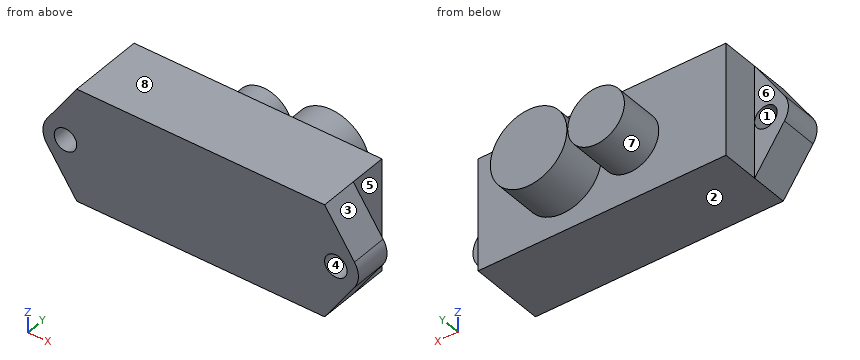
```python
from build123d import *

# Parameters (mm, degrees)
BOSS_EXTRUDE11_DEPTH   = 5
BOSS_EXTRUDE11_2_DEPTH = 5
SKETCH1_5_W            = 33
SKETCH1_5_H            = 15
BOSS_EXTRUDE13_DEPTH   = 10
SKETCH2_R              = 1.5
CUT_EXTRUDE1_DEPTH     = 5
SKETCH3_R              = 3.777846651
BOSS_EXTRUDE18_DEPTH   = 6
SKETCH3_5_R            = 5.1
BOSS_EXTRUDE22_DEPTH   = 6


with BuildPart() as part:
    # Sketch1 → Boss-Extrude11 (new body)
    with BuildSketch(Plane(origin=(0, 0, 0), x_dir=(1, 0, 0), z_dir=(0, 1, 0))):
        with BuildLine():
            Line((-20.475239861, 1.695047972), (-16.5, 7.5))
            Line((-16.5, 7.5), (-16.5, -7.5))
            Line((-16.5, -7.5), (-20.475239861, -1.695047972))
            ThreePointArc((-20.475239861, -1.695047972), (-21, 0), (-20.475239861, 1.695047972))
        make_face()
    extrude(amount=BOSS_EXTRUDE11_DEPTH)



with BuildPart() as body_2:
    # Sketch1 → Boss-Extrude11 2 (new body)
    with BuildSketch(Plane(origin=(0, 0, 0), x_dir=(1, 0, 0), z_dir=(0, 1, 0))):
        with BuildLine():
            ThreePointArc((20.475239861, 1.695047972), (21, 0), (20.475239861, -1.695047972))
            Line((20.475239861, -1.695047972), (16.5, -7.5))
            Line((16.5, -7.5), (16.5, 7.5))
            Line((16.5, 7.5), (20.475239861, 1.695047972))
        make_face()
    extrude(amount=BOSS_EXTRUDE11_2_DEPTH)


with BuildPart() as part_1:
    add(part.part)

    add(body_2.part)  # Boss-Extrude13 merges body 2
    # Sketch1_5 → Boss-Extrude13 (add)
    with BuildSketch(Plane(origin=(0, 0, 0), x_dir=(1, 0, 0), z_dir=(0, 1, 0))):
        Rectangle(SKETCH1_5_W, SKETCH1_5_H)
    extrude(amount=BOSS_EXTRUDE13_DEPTH)

    # Sketch2 → Cut-Extrude1 (cut)
    with BuildSketch(Plane(origin=(0, 5, 0), x_dir=(1, 0, 0), z_dir=(0, 1, 0))):
        with Locations(Location((-18, 0, 0), (0, 0, 270))):
            Circle(SKETCH2_R)
        with Locations(Location((18, 0, 0), (0, 0, 270))):
            Circle(SKETCH2_R)
    extrude(amount=-CUT_EXTRUDE1_DEPTH, mode=Mode.SUBTRACT)

    # Sketch3 → Boss-Extrude18 (add)
    with BuildSketch(Plane(origin=(0, 10, 0), x_dir=(1, 0, 0), z_dir=(0, 1, 0))):
        with Locations(Location((-3.777846651, 0, 0), (0, 0, 270))):
            Circle(SKETCH3_R)
    extrude(amount=BOSS_EXTRUDE18_DEPTH)

    # Sketch3_5 → Boss-Extrude22 (add)
    with BuildSketch(Plane(origin=(0, 10, 0), x_dir=(1, 0, 0), z_dir=(0, 1, 0))):
        with Locations(Location((5.2, 0, 0), (0, 0, 270))):
            Circle(SKETCH3_5_R)
    extrude(amount=BOSS_EXTRUDE22_DEPTH)


solid = part_1.part
```
For this review, take the finished solid that the model builds, in its own axes (mm). Face numbers are marked on the shaded views. A direction names the side the tool comes from. Round coordinates to 2 decimals unless told otherwise and drop trailing zeros. Write each loop counter-clockwise with the first axis right and the second up, starting at its lowest first coordinate (ties: lowest second). Pieces come first, ordered by that corner, then holes. Notation, with made-up numbers: (24, -17.75) - (39, -17.75) arc R22 cw to (39, 3.25) - close; hole circle Ø4 at (75.5, 15.25). An arc over 180 degrees is marked (long way). Answer as a JSON object with one key per item and string values.
1. We need section D-D on y = 12.5. Give the boundary of the cut face in (x, z).
Response values:
{"outline": "circle Ø7.56 at (-3.78, 0); circle Ø10.2 at (5.2, 0)"}
2. We need section B-B on z = 0.5. Give the boundary of the cut face in (x, y).
Response values:
{"outline": "(-20.96, 0) - (-19.41, 0) - (-19.41, 5) - (-20.96, 5) - close; (-16.59, 0) - (16.59, 0) - (16.59, 5) - (16.5, 5) - (16.5, 10) - (10.28, 10) - (10.28, 16) - (0.12, 16) - (0.12, 10) - (-0.03, 10) - (-0.03, 16) - (-7.52, 16) - (-7.52, 10) - (-16.5, 10) - (-16.5, 5) - (-16.59, 5) - close; (19.41, 0) - (20.96, 0) - (20.96, 5) - (19.41, 5) - close"}
3. We need section A-A on y = 1. Give the boundary of the cut face in (x, z), then the cut area to 3 significant figures.
Response values:
{"outline": "(-20.48, -1.7) - (-16.5, -7.5) - (16.5, -7.5) - (20.48, -1.7) arc R3 ccw to (20.48, 1.7) - (16.5, 7.5) - (-16.5, 7.5) - (-20.48, 1.7) arc R3 ccw to start; hole circle Ø3 at (-18, 0); hole circle Ø3 at (18, 0)", "area": "556 mm2"}
4. For pin 1 Ø3.5 at (x, z) = (18, 1) entering from +Y; pin 2 Ø1.5 at (y, z) = (8.5, -0.5) entering from -X; pin 3 Ø6 at (y, z) = (9, 2) entering from +X, all flat-tipped, find the tip position at first contact; note any pin that passes through.
Response values:
{"pin 1": "stops at y = 10", "pin 2": "stops at x = -16.5", "pin 3": "stops at x = 16.5"}
5. To check wall thickness, follow line 1 along X through (y, z) = (1.6, 0); line 2 along Y through (x, z) = (-13.5, 6.75); line 3 along Z through (x, y) = (-18, 3.2). State the ranges of each line that lie inside material, in increasing order.
Response values:
{"line 1": "x = -21 to -19.5, -16.5 to 16.5, 19.5 to 21", "line 2": "y = 0 to 10", "line 3": "z = -5.31 to -1.5, 1.5 to 5.31"}
6. Tool access review of the marked faces 4, 5, 6, 7 and 8: name each direction out of +Z, -Z, +X, -X, +Y, -Y from which nothing blocks a thin tool from reaching the whole face with its end or side.
Response values:
{"face 4": "+Y, -Y", "face 5": "+Z, -Z, +X, +Y", "face 6": "+Z, -Z, -X, +Y", "face 7": "+Y", "face 8": "+Z, +X, -X, +Y, -Y"}
7. We need section C-C on x = -18. Give the boundary of the cut face in (y, z), then the cut area to 3 significant figures.
Response values:
{"outline": "(0, -5.31) - (5, -5.31) - (5, -1.5) - (0, -1.5) - close; (0, 1.5) - (5, 1.5) - (5, 5.31) - (0, 5.31) - close", "area": "38.1 mm2"}
8. Draft analysis for pull direction Z (two halves, no side actions). For the marked faces 1, 2 and 3, state which applies: +Z half, -Z half, draft (parallel to the pull), parting line (faces both ways), or undercut.
Response values:
{"face 1": "undercut", "face 2": "-Z half", "face 3": "+Z half"}
